Autodesk Inventor part; units mm, degrees
ref_plane "YZ Plane" through (0, 0, 0) normal (1, 0, 0) x (0, 1, 0)
ref_plane "XZ Plane" through (0, 0, 0) normal (0, 1, 0) x (-1, 0, 0)
ref_plane "XY Plane" through (0, 0, 0) normal (0, 0, 1) x (1, 0, 0)
sketch "Sketch1" plane through (0, 0, 0) normal (0, 1, 0) x (-1, 0, 0)
  line L0 (0, 0) -> (-15, 0)
  line L1 (-15, 0) -> (-15, -14)
  line L2 (-15, -14) -> (0, -14)
  line L3 (0, -14) -> (0, 0)
  line L4 (0, -4.2) -> (-15, -4.2)
  line L5 (-3, 0) -> (-3, -14)
  circle A0 centre (-4.25, -5.45) radius 1.25
  line L6 (-12, -2) -> (-14, -2)
  line L7 (-14, -2) -> (-14, -12)
  line L8 (-14, -12) -> (-12, -12)
  line L9 (-12, -12) -> (-12, -2)
  line L10 (-12, -2) -> (-8.5, -2)
  line L11 (-8.5, -2) -> (-8.5, -4.6)
  line L12 (-8.5, -4.6) -> (-12, -4.6)
  line L13 (-12, -4.6) -> (-12, -2)
  line L14 (-12, -12) -> (-8.5, -12)
  line L15 (-8.5, -12) -> (-8.5, -9.4)
  line L16 (-8.5, -9.4) -> (-12, -9.4)
  line L17 (-12, -9.4) -> (-12, -12)
  dimension "d0" = 15
  dimension "d1" = 14
  dimension "d2" = 4.2
  dimension "d3" = 3
  dimension "d4" = 2.5
  dimension "d5" = 10
  dimension "d6" = 2
  dimension "d7" = 2
  dimension "d8" = 2
  dimension "d9" = 1
  dimension "d10" = 3.5
  dimension "d11" = 3.5
  dimension "d12" = 2.6
  dimension "d13" = 2.6
  dimension "d14" = 2
  dimension "d15" = 2
extrude "Extrusion1" add sketch "Sketch1" against normal blind 0.8 contours L3 L4 L5 L0 | L5 L4 L11 L10 L6 L7 L1 L0 | L3 L2 L5 L4 | L5 A0 L4 | L4 L7 L8 L14 L15 L16 L9 L12 L11 A0 L5 L2 L1 | L7 L6 L9 L4 | L4 L9 L8 L7 | L11 L12 L9 L4 | L4 L9 L10 L11 | L9 L16 L15 L14
extrude "Extrusion2" add sketch "Sketch1" along normal blind 1.2 contours L11 L12 L9 L4 | L4 L9 L10 L11 | L9 L16 L15 L14
extrude "Extrusion3" add sketch "Sketch1" against normal blind 1.8 contours L7 L6 L9 L4 | L4 L9 L8 L7
equation "\"d7\" = d8"
properties part number "line_sensor" material "Thermoplastic Resin"
Input: part model. Units: mm. Frame: model coordinates. A direction names the side the tool comes from. Coordinates: 2 decimals unless noted, no trailing zeros. Order: outer loops, then holes, each group sorted by start corner. A loop starts at its lowest first (then second) coordinate and runs counter-clockwise, first axis right, second up.
1. Access query for faces 5 (the flat face through (14, -1, -7)), 6 (the flat face through (12, 1, -11)), 7 (the flat face through (8.5, 1, -3)), 8 (the flat face through (10, 1, -2)). Directions: +Z, -Z, +X, -X, +Y, -Y. A direction counts if a zero-diameter tool reaches every point of the face in a straight line with its end or side. Return the directions, or none.
Checked values:
face 5: +Z, -Z, +X, -Y
face 6: +Z, -Z, +X, +Y
face 7: +Z, -Z, -X, +Y
face 8: +Z, +X, -X, +Y
2. Draft query along Z for faces 1 (the flat face through (10, 1, -4.6)), 2 (the flat face through (10, 1, -9.4)), 3 (the flat face through (12, -1, -7)), 4 (the flat face through (13, -1, -12)). Return one class per face: +Z half, -Z half, draft (parallel to the pull), parting line (faces both ways), or undercut.
Checked values:
face 1: undercut
face 2: undercut
face 3: draft
face 4: -Z half
3. Cut plane B-B, the plane z = -5.45. Return loops of the section in (x, y), plus the area to 3 significant figures.
Checked values:
outline: (0, -0.8) - (3, -0.8) - (3, 0) - (0, 0) - close; (5.5, -0.8) - (12, -0.8) - (12, -1.8) - (14, -1.8) - (14, -0.8) - (15, -0.8) - (15, 0) - (5.5, 0) - close
area: 12.0 mm2
4. Contact query for flat-ended pins moving along their axis: P1, Ø4, axis at x = 4.5, z = -5.5, coming from the +Y side; P2, Ø0.5, axis at y = -1.5, z = -5, coming from the -X side; P3, Ø0.6, axis at y = 0.5, z = -10.5, coming from the -X side; P4, Ø1.1, axis at x = 12.5, y = -1, coming from the -Z side. Output: stop coordinate, or through.
Checked values:
P1: stops at y = 0
P2: stops at x = 12
P3: stops at x = 8.5
P4: stops at z = -14
5. Cut plane A-A, the plane y = 0.8. Return loops of the section in (x, z).
Checked values:
outline: (8.5, -12) - (12, -12) - (12, -9.4) - (8.5, -9.4) - close; (8.5, -4.6) - (12, -4.6) - (12, -2) - (8.5, -2) - close
6. Cut plane C-C, the plane x = 4.25. Return loops of the section in (y, z), plus the area to 3 significant figures.
Checked values:
outline: (-0.8, -14) - (0, -14) - (0, -6.7) - (-0.8, -6.7) - close; (-0.8, -4.2) - (0, -4.2) - (0, 0) - (-0.8, 0) - close
area: 9.20 mm2
7. Ray query, line 1 along Z through (x, y) = (4.25, -0.45); line 2 along X through (y, z) = (-0.3, -5.45); line 3 along Z through (x, y) = (9.5, 0.05). Return the intervals inside material, ascending.
Checked values:
line 1: z = -14 to -6.7, -4.2 to 0
line 2: x = 0 to 3, 5.5 to 15
line 3: z = -12 to -9.4, -4.6 to -2
8. Cut plane D-D, the plane y = -0.35. Return loops of the section in (x, z), plus the area to 3 significant figures.
Checked values:
outline: (0, -14) - (15, -14) - (15, 0) - (0, 0) - close; hole circle Ø2.5 at (4.25, -5.45)
area: 205 mm2
